```python
from build123d import *

# Parameters (mm, degrees)
F0_R      = 4.9
F1_DEPTH  = 18
F1_FACE_R = 4.9
F3_R      = 10
F5_R      = 1.5
F6_DEPTH  = 15
F7_R      = 4
F8_DEPTH  = 17.5


with BuildPart() as f1:
    # F0 (on Front) → F1 (new body)
    with BuildSketch(Plane.XZ):
        Circle(F0_R)
    extrude(amount=F1_DEPTH)

    # F1_face (on face) → F4 section 0
    with BuildSketch(Plane.XZ.offset(18)):
        Circle(F1_FACE_R)
    # F3 (on offset) → F4 section 1
    with BuildSketch(Plane.XZ.offset(30)):
        Circle(F3_R)
    loft()

    # F5 (on face) → F6 (cut)
    with BuildSketch(Plane(origin=(0, 0, 0), x_dir=(-1, 0, 0), z_dir=(0, 1, 0))):
        Circle(F5_R)
    extrude(amount=-F6_DEPTH, mode=Mode.SUBTRACT)

    # F7 (on face) → F8 (cut)
    with BuildSketch(Plane.XZ.offset(30)):
        Circle(F7_R)
    extrude(amount=-F8_DEPTH, mode=Mode.SUBTRACT)


solid = f1.part
```
Geometry: final body of the model. Coordinates: model frame, mm. A direction names the side the tool comes from. Give positions to 0.01 mm unless a question says otherwise; leave off trailing zeros. Order: outer loops, then holes, each group sorted by start corner. A loop starts at its lowest first (then second) coordinate and runs counter-clockwise, first axis right, second up. Notation, with made-up numbers: (44.25, -4.5) -> (63.25, -4.5) arc R12 ccw to (63.25, 4.5) -> close; hole circle Ø3 at (-15, 77). An arc over 180 degrees is marked (long way). Write each question's results on one line, items separated by ' | '. Start each with the question number.
1) Section C-C (y = -5.5). Return loops of the section in (x, z).
2) First-contact query: pin 1 (6 mm diameter, centred on y = -8, z = -6.5, fed in from +X); pin 2 (4 mm diameter, centred on y = -15, z = -4.5, fed in from -X); pin 3 (12 mm diameter, centred on x = -7, y = -7.5, fed in from +Z); pin 4 (2 mm diameter, centred on y = -18.5, z = -7, fed in from -X). Flat tips, straight axial feed; report the tip coordinate or a pass-through.
3) Line query: line 1 (Z direction, x = 0, y = -8); line 2 (Y direction, x = -3.5, z = 0); line 3 (X direction, y = -22, z = -2.75). Output: solid intervals per line, ascending. Write a range as from..to.
4) Set-up query: faces 1 (the cylindrical face through (-1.062, -8.874, -4.783)), 2 (the flat face through (-1.2, 0, 1.2)), 3 (the cylindrical face through (-0.867, -21.373, -3.905)). Return all of +Z, -Z, +X, -X, +Y, -Y with unobstructed straight access to the full face (end or side cutting, diameter ignored); none if empty.
5) Section B-B (y = -17). Return loops of the section in (x, z), then the cut area to 3 significant figures.
6) Section A-A (x = 0). Return loops of the section in (y, z).
7) Draft query along X for faces 4 (the flat face through (4.3, -30, 0.1)), 5 (the conical face through (-1.38, -21.42, -6.2)), 6 (the flat face through (2, -12.5, 0)). Return one class per face: pulls with the +X half, pulls with the -X half, needs draft (parallel to the pull), parting line crosses it, or undercut.
Calculated:
1) outline: circle Ø9.8 at (0, 0); hole circle Ø3 at (0, 0)
2) pin 1: x = 3.43 | pin 2: x = -4.21 | pin 3: z = 4.8 | pin 4: through
3) line 1: -4.9..-1.5, 1.5..4.9 | line 2: -12.5..0 | line 3: -6..-2.9, 2.9..6
4) face 1: +Y | face 2: +Z, -Z, +X, -X, +Y | face 3: -Y
5) outline: circle Ø9.8 at (0, 0); hole circle Ø8 at (0, 0) | area: 25.2 mm2
6) outline: (-30, -10) -> (-18, -4.9) -> (0, -4.9) -> (0, -1.5) -> (-12.5, -1.5) -> (-12.5, -4) -> (-30, -4) -> close; (-30, 4) -> (-12.5, 4) -> (-12.5, 1.5) -> (0, 1.5) -> (0, 4.9) -> (-18, 4.9) -> (-30, 10) -> close
7) face 4: needs draft | face 5: parting line crosses it | face 6: undercut
